from build123d import *

# Parameters (mm, degrees)
SKETCH1_W                  = 5
SKETCH1_H                  = 15
SKETCH2_R                  = 7.5
BOSS_EXTRUDE1_DEPTH        = 15
F_4_3_4_3_DIAMETER_HOLE1_D = 4.3
F_6_5_6_5_DIAMETER_HOLE1_D = 6.5
CHAMFER1_SIZE              = 0.75
CHAMFER2_SIZE              = 0.5
FILLET1_R                  = 0.4


with BuildPart() as part:
    # Sketch1 → Revolve1 (revolve)
    with BuildSketch(Plane(origin=(0, 0, 0), x_dir=(-1, 0, 0), z_dir=(0, 0, -1)), mode=Mode.PRIVATE) as revolve1_sk:
        with Locations((-2.5, 7.5)):
            Rectangle(SKETCH1_W, SKETCH1_H)
    revolve(revolve1_sk.sketch.rotate(Axis((5, 0, 0), (-1, 0, 0)), 270), axis=Axis((5, 0, 0), (-1, 0, 0)))

    # Sketch2 → Boss-Extrude1 (add)
    with BuildSketch(Plane(origin=(5, 0, 0), x_dir=(0, 0, -1), z_dir=(1, 0, 0))):
        Circle(SKETCH2_R)
    extrude(amount=BOSS_EXTRUDE1_DEPTH)

    # Ø4.3 (4.3) Diameter Hole1 (through all)
    with Locations(Plane(origin=(5, 0, 0), x_dir=(0, 0, -1), z_dir=(1, 0, 0))):
        with Locations((-11, 0), (11, 0), (0, -11), (0, 11)):
            Hole(F_4_3_4_3_DIAMETER_HOLE1_D / 2)

    # Ø6.5 (6.5) Diameter Hole1 (through all)
    with Locations(Plane.ZY):
        with Locations((0, 0)):
            Hole(F_6_5_6_5_DIAMETER_HOLE1_D / 2)

    # Chamfer1
    chamfer1_edges = [part.edges().sort_by_distance(p)[0] for p in [
        (0, 0, 3.25),
        (20, 0, 3.25),
    ]]
    chamfer(chamfer1_edges, length=CHAMFER1_SIZE)

    # Chamfer2
    chamfer2_edges = [part.edges().sort_by_distance(p)[0] for p in [
        (0, 0, -15),
        (5, 0, -15),
        (20, 0, 7.5),
    ]]
    chamfer(chamfer2_edges, length=CHAMFER2_SIZE)

    # Fillet1
    fillet1_edges = [part.edges().sort_by_distance(p)[0] for p in [
        (5, 0, 7.5),
    ]]
    fillet(fillet1_edges, radius=FILLET1_R)


solid = part.part
Geometry check sheet. Reference: the model listing, model coordinates, mm. Give positions to 0.01 mm unless a question says otherwise; leave off trailing zeros. Order: outer loops, then holes, each group sorted by start corner. A loop starts at its lowest first (then second) coordinate and runs counter-clockwise, first axis right, second up.
1) Draft check along Z on faces 1 (the cylindrical face through (12.351, 0.33, 7.493)), 2 (the flat face through (5, -6, -6)), 3 (the cylindrical face through (2.46, 0.65, -8.95)), 4 (the cylindrical face through (2.465, 9.692, -1.706)). Enter one of: released by +Z, released by -Z, zero draft, split by the parting line, or undercut.
Results are:
face 1: split by the parting line
face 2: zero draft
face 3: undercut
face 4: undercut
2) Gauge pin test, flat ends, axial feed: pin 1 (1.5 mm diameter, centred on x = 11, y = 6.5, fed in from +Z); pin 2 (2 mm diameter, centred on x = 9, z = -1, fed in from -Y); pin 3 (1.5 mm diameter, centred on x = 5, z = 1.5, fed in from +Y). Record the tip position at first contact, or that the pin passes through.
Results are:
pin 1: stops at z = 4.82
pin 2: stops at y = -7.5
pin 3: stops at y = 14.97
3) Material ranges on probe 1 along Y at (x, z) = (3.95, 0); probe 2 along Y at (x, z) = (12.5, 0); probe 3 along X at (y, z) = (-8, 8.5), recorded low to high.
Results are:
probe 1: y = -15 to -13.15, -8.85 to -3.25, 3.25 to 8.85, 13.15 to 15
probe 2: y = -7.5 to -3.25, 3.25 to 7.5
probe 3: x = 0 to 5
4) Cross-section at C-C (x = 11.5). Record the boundary of the cut face in (y, z).
Results are:
outline: circle Ø15 at (0, 0); hole circle Ø6.5 at (0, 0)
5) Cross-section at A-A (y = 0). Give the number of separate pieces and of enclosed holes in the cut face, then the cut area to 3 significant figures.
Results are:
separate pieces: 4
enclosed holes: 0
area: 200 mm2
